The listing builds one solid part. Answer for the finished solid, in the listing's coordinates (mm). Face numbers are marked on the shaded views. A direction names the side the tool comes from. Coordinates: 2 decimals unless noted, no trailing zeros. Write each loop counter-clockwise with the first axis right and the second up, starting at its lowest first coordinate (ties: lowest second). Pieces come first, ordered by that corner, then holes.
Autodesk Inventor part; units mm, degrees
ref_plane "YZ Plane" through (0, 0, 0) normal (1, 0, 0) x (0, 1, 0)
ref_plane "XZ Plane" through (0, 0, 0) normal (0, 1, 0) x (-1, 0, 0)
ref_plane "XY Plane" through (0, 0, 0) normal (0, 0, 1) x (1, 0, 0)
sketch "Sketch1" plane through (0, 0, 0) normal (0, 1, 0) x (-1, 0, 0)
  line L0 (0, -2.5) -> (-2.1651, -1.25)
  line L1 (-2.1651, -1.25) -> (-2.1651, 1.25)
  line L2 (-2.1651, 1.25) -> (0, 2.5)
  line L3 (0, 2.5) -> (2.1651, 1.25)
  line L4 (2.1651, 1.25) -> (2.1651, -1.25)
  line L5 (2.1651, -1.25) -> (0, -2.5)
  point P0 (0, 0)
  point P1 (0, 0)
  dimension "d0" = 5
extrude "Extrusion1" add sketch "Sketch1" along normal blind 1.5
sketch "Sketch2" plane through (0, 1.5, 0) normal (0, 1, 0) x (1, 0, 0)
  circle A0 centre (0, 0) radius 1.25
  dimension "d3" = 2.5
extrude "Extrusion2" add sketch "Sketch2" along normal blind 2.5
thread "Thread1"
sketch "Sketch3" plane through (0, 4, 0) normal (0, 1, 0) x (1, 0, 0)
  circle A0 centre (0, 0) radius 0.75
  dimension "d10" = 1.5
extrude "Extrusion3" add sketch "Sketch3" along normal blind 1.5
properties material "Steel, Mild"
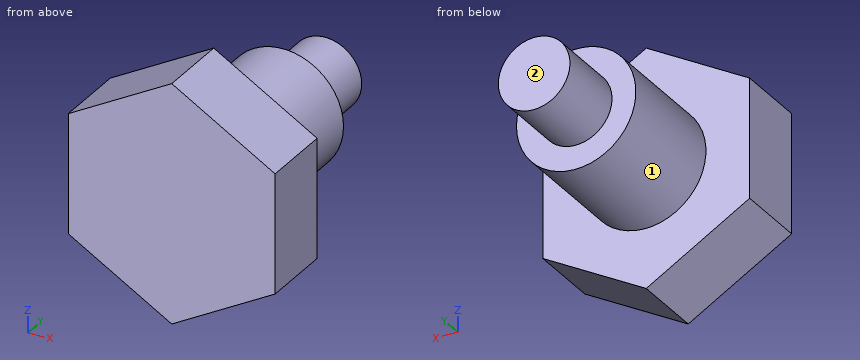
1. Section D-D on y = 4.8 is taken. Give the vertices of the cut face in (x, z), then the cut area to 3 significant figures.
Results found:
outline: circle Ø1.5 at (0, 0)
area: 1.77 mm2
2. Section B-B on y = 1 is taken. Give the vertices of the cut face in (x, z).
Results found:
outline: (-2.17, -1.25) - (0, -2.5) - (2.17, -1.25) - (2.17, 1.25) - (0, 2.5) - (-2.17, 1.25) - close
3. Section C-C on x = -0.5 is taken. Give the vertices of the cut face in (y, z), then the cut area to 3 significant figures.
Results found:
outline: (0, -2.21) - (1.5, -2.21) - (1.5, -1.15) - (4, -1.15) - (4, -0.56) - (5.5, -0.56) - (5.5, 0.56) - (4, 0.56) - (4, 1.15) - (1.5, 1.15) - (1.5, 2.21) - (0, 2.21) - close
area: 14.0 mm2
4. Section A-A on z = 0 is taken. Give the vertices of the cut face in (x, y), then the cut area to 3 significant figures.
Results found:
outline: (-2.17, 0) - (2.17, 0) - (2.17, 1.5) - (1.25, 1.5) - (1.25, 4) - (0.75, 4) - (0.75, 5.5) - (-0.75, 5.5) - (-0.75, 4) - (-1.25, 4) - (-1.25, 1.5) - (-2.17, 1.5) - close
area: 15.0 mm2
5. Find the intervals of material crossed by L1, parallel to Y at x = -1.45, z = -0.15; L2, parallel to Y at x = 1.1, z = -0.4; L3, parallel to X at y = 5.2, z = 0, in increasing order.
Results found:
L1: y = 0 to 1.5
L2: y = 0 to 4
L3: x = -0.75 to 0.75
6. Flat-ended cylindrical pins translate along their axes: P1, Ø1.5, axis at y = 4, z = -1, coming from the +X side; P2, Ø3, axis at y = 4, z = -1, coming from the -X side. Find the tip coordinate at first contact, or state that the pin passes through.
Results found:
P1: stops at x = 1.22
P2: stops at x = -1.25
7. A tool of negligible diameter and unlimited length cuts with its end or side. For the marked faces 1 and 2, from which of +Z, -Z, +X, -X, +Y, -Y can it reach the whole face along a straight path? Write none if from no direction.
Results found:
face 1: +Y
face 2: +Z, -Z, +X, -X, +Y
